Work out the finished part from the listing and answer in its coordinate system (mm). Round coordinates to 2 decimals unless told otherwise and drop trailing zeros. Write each loop counter-clockwise with the first axis right and the second up, starting at its lowest first coordinate (ties: lowest second). Pieces come first, ordered by that corner, then holes. Notation, with made-up numbers: (81, 78.5) - (136, 78.5) arc R22 cw to (136, 110.5) - close; hole circle Ø6 at (0.25, 52). An arc over 180 degrees is marked (long way). Answer as a JSON object with one key per item and string values.
Autodesk Fusion 360 part; units mm, degrees
sketch "Esboço1" plane through (0, 0, 0) normal (0, 0, 1) x (1, 0, 0)
  line L0 (18.163, 18) -> (75.223, 18)
  line L1 (75.223, 18) -> (75.223, 12)
  line L2 (75.223, 12) -> (18.163, 12)
  line L3 (18.163, 12) -> (18.163, 18)
  circle A0 centre (22.163, 15) radius 1.6
  circle A1 centre (71.223, 15) radius 1.6
  dimension "d2" = 3.2
  dimension "d3" = 3.2
  dimension "d4" = 49.06
  dimension "d5" = 4
  dimension "d6" = 4
  dimension "d13" = 6
  dimension "d14" = 3
extrude "Extrusão1" add sketch "Esboço1" along normal blind 4
fillet "Arredondamento3" radius 3 2 edges at (18.163, 18, 2) (18.163, 12, 2)
fillet "Arredondamento4" radius 3 2 edges at (75.223, 18, 2) (75.223, 12, 2)
scale "Escala1" factor 0.7 about (20.563, 15, 0) bodies 1
scale "Escala2" factor 1.14 about (20.983, 17.1, 2.8) bodies 1
Item 1: Each of these flat-tipped pins is pushed along its axis until it touches: P1, Ø1.5, axis at y = 13, z = 2, coming from the +X side; P2, Ø1, axis at y = 14, z = 1.5, coming from the -X side. Where does it stop, or does it pass through?
Results found:
{"P1": "x = 63.92", "P2": "x = 18.6"}
Item 2: A cutting plane is placed at B-B (y = 16.5). Write down the section's boundary in (x, z).
Results found:
{"outline": "(19.4, -0.39) - (63.31, -0.39) - (63.31, 2.8) - (19.4, 2.8) - close"}
Item 3: A cutting plane is placed at C-C (y = 12.8). Write down the section's boundary in (x, z), and give its area (3 significant figures).
Results found:
{"outline": "(19.53, -0.39) - (63.18, -0.39) - (63.18, 2.8) - (19.53, 2.8) - close", "area": "139 mm²"}
Item 4: Determine the mould class of faces 1 (the cylindrical face through (19.272, 13.032, 1.226)), 2 (the cylindrical face through (62.11, 15.2, 1.18)), 3 (the cylindrical face through (63.44, 16.38, 1.23)) for opening direction X: pulls with the +X half, pulls with the -X half, needs draft (parallel to the pull), parting line crosses it, or undercut.
Results found:
{"face 1": "pulls with the -X half", "face 2": "undercut", "face 3": "pulls with the +X half"}
Item 5: Consider line 1 along X through (y, z) = (14.6, 1.7); line 2 along X through (y, z) = (15, 1.5); line 3 along Y through (x, z) = (60.5, 0.7). Determine where each line is inside the solid, lowest interval first.
Results found:
{"line 1": "18.59 to 20.51, 23.05 to 59.66, 62.2 to 64.12", "line 2": "18.61 to 20.54, 23.02 to 59.69, 62.17 to 64.1", "line 3": "12.31 to 13.5, 15.91 to 17.1"}
Item 6: A cutting plane is placed at A-A (z = 2.05). Give the number of separate pieces and of enclosed holes in the cut face, and give its area (3 significant figures).
Results found:
{"separate pieces": "1", "enclosed holes": "2", "area": "203 mm²"}
